Can you work these out from the model? Positions are in its coordinate system, mm. Face numbers are marked on the shaded views. A direction names the side the tool comes from. Coordinates: 2 decimals unless noted, no trailing zeros. Order: outer loops, then holes, each group sorted by start corner. A loop starts at its lowest first (then second) coordinate and runs counter-clockwise, first axis right, second up. Notation, with made-up numbers: (-13.75, 30) -> (0.25, 30) arc R13 ccw to (0.25, 47) -> close; hole circle Ø8 at (86.5, 28.25). An arc over 180 degrees is marked (long way). Answer as CSV lines item,"result".
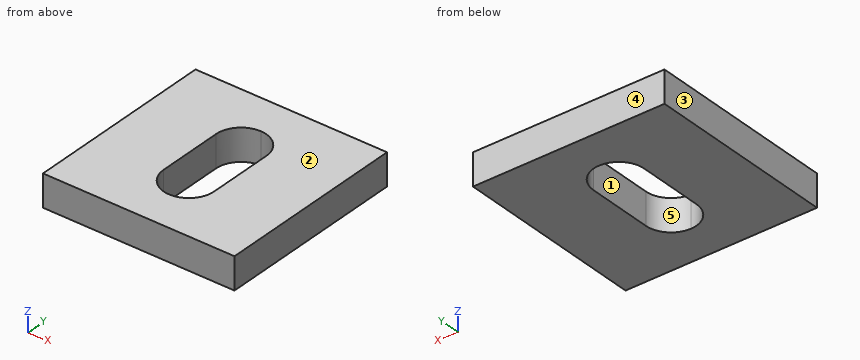
from build123d import *

# Parameters (mm, degrees)
F0_W     = 19
F0_H     = 19
F0_W_2   = 5
F0_H_2   = 11.5
F1_DEPTH = 3.175
F2_R     = 2.49999


# Not quite as in the source:
# - a fillet or chamfer is up to 0.001 mm smaller than in the source, because OpenCascade refuses the exact size


with BuildPart() as f1:
    # F0 (on Top) → F1 (new body)
    with BuildSketch(Plane.XY):
        Rectangle(F0_W, F0_H)
        Rectangle(F0_W_2, F0_H_2, mode=Mode.SUBTRACT)
    extrude(amount=F1_DEPTH)

    # F2 (radius 2.5 in the source; OpenCascade refuses exactly that, so slightly less here)
    f2_edges = [f1.edges().sort_by_distance(p)[0] for p in [
        (-2.5, 5.75, 1.5875),
        (-2.5, -5.75, 1.5875),
        (2.5, 5.75, 1.5875),
        (2.5, -5.75, 1.5875),
    ]]
    fillet(f2_edges, radius=F2_R)


solid = f1.part
Q1. If I drill on line 1 (X direction, y = -2, z = 1.8); line 2 (Y direction, x = 0.5, z = 0.3); line 3 (X direction, y = 4, z = 0.85), over which ranges is the centre line in solid material (lowest first)?
Solution:
line 1,"-9.5 to -2.5, 2.5 to 9.5"
line 2,"-9.5 to -5.7, 5.7 to 9.5"
line 3,"-9.5 to -2.38, 2.38 to 9.5"
Q2. Imagine slicing it at A-A (y = 3). List the corners of the cut face in (x, z) for me (3 decimals).
Solution:
outline,"(-9.5, 0) -> (-2.5, 0) -> (-2.5, 3.175) -> (-9.5, 3.175) -> close; (2.5, 0) -> (9.5, 0) -> (9.5, 3.175) -> (2.5, 3.175) -> close"
Q3. We'd pull the mould along Y, two halves only. Please class the marked faces 3, 4 and 5: pulls with the +Y half, pulls with the -Y half, needs draft (parallel to the pull), parting line crosses it, or undercut.
Solution:
face 3,"needs draft"
face 4,"pulls with the +Y half"
face 5,"undercut"
Q4. Imagine slicing it at C-C (x = 1.75). List the corners of the cut face in (y, z) for me (3 decimals), and give its area (3 significant figures).
Solution:
outline,"(-9.5, 0) -> (-5.035, 0) -> (-5.035, 3.175) -> (-9.5, 3.175) -> close; (5.035, 0) -> (9.5, 0) -> (9.5, 3.175) -> (5.035, 3.175) -> close"
area,"28.4 mm2"
Q5. Which directions (+Z, -Z, +X, -X, +Y, -Y) give clear straight access to the entire face, cutting with the end or side of a thin tool? Please do the marked faces 1 and 2.
Solution:
face 1,"+Z, -Z"
face 2,"+Z, +X, -X, +Y, -Y"
